```python
from build123d import *

# Parameters (mm, degrees)
SKETCH1_W           = 40
SKETCH1_H           = 30
BOSS_EXTRUDE1_DEPTH = 2
SKETCH2_W           = 20
SKETCH2_H           = 30
BOSS_EXTRUDE2_DEPTH = 2
SKETCH3_W           = 20
SKETCH3_H           = 30
BOSS_EXTRUDE3_DEPTH = 2
SKETCH5_R           = 5
CUT_EXTRUDE2_DEPTH  = 55.595167513


with BuildPart() as part:
    # Sketch1 → Boss-Extrude1 (new body)
    with BuildSketch(Plane.XY):
        with Locations((-21.168831169, 10.38961039)):
            Rectangle(SKETCH1_W, SKETCH1_H)
    extrude(amount=BOSS_EXTRUDE1_DEPTH)

    # Sketch2 → Boss-Extrude2 (add)
    with BuildSketch(Plane.ZY.offset(41.168831169)):
        with Locations((10, 10.38961039)):
            Rectangle(SKETCH2_W, SKETCH2_H)
    extrude(amount=BOSS_EXTRUDE2_DEPTH)

    # Sketch3 → Boss-Extrude3 (add)
    with BuildSketch(Plane(origin=(-1.168831169, 0, 0), x_dir=(0, 0, -1), z_dir=(1, 0, 0))):
        with Locations((-10, 10.38961039)):
            Rectangle(SKETCH3_W, SKETCH3_H)
    extrude(amount=BOSS_EXTRUDE3_DEPTH)

    # Sketch5 → Cut-Extrude2 (cut, through all)
    with BuildSketch(Plane(origin=(0.831168831, 0, 0), x_dir=(0, 0, -1), z_dir=(1, 0, 0))):
        with Locations(Location((-10, 10.38961039, 0), (0, 0, 90))):
            Circle(SKETCH5_R)
    extrude(amount=-CUT_EXTRUDE2_DEPTH, mode=Mode.SUBTRACT)


solid = part.part
```
Model file for the job. Use its own axes, mm. A direction names the side the tool comes from. Give positions to 0.01 mm unless a question says otherwise; leave off trailing zeros. Write each loop counter-clockwise with the first axis right and the second up, starting at its lowest first coordinate (ties: lowest second). Pieces come first, ordered by that corner, then holes. Notation, with made-up numbers: M -1.5,4.25 L 35.5,4.25 A17 cw 35.5,36.25 Z; hole C 83.25,45 d9. An arc over 180 degrees is marked long. Use a Markdown table: item, result.
1) Cut at D-D (y = 23.75). List the corners of the cut face in (x, z).
Responses:
| item | result |
|---|---|
| outline | M -43.17,0 L 0.83,0 L 0.83,20 L -1.17,20 L -1.17,2 L -41.17,2 L -41.17,20 L -43.17,20 Z |
2) Drill centre lines: line 1 (X direction, y = 15.75, z = 18.75); line 2 (Z direction, x = -41, y = 11.5). Where is each one in solid material? Low to high. Write a range as from..to.
Responses:
| item | result |
|---|---|
| line 1 | x = -43.17..-41.17, -1.17..0.83 |
| line 2 | z = 0..2 |
3) Cut at B-B (y = 7.75). List the corners of the cut face in (x, z), and give its area (3 significant figures).
Responses:
| item | result |
|---|---|
| outline | M -43.17,0 L 0.83,0 L 0.83,5.75 L -1.17,5.75 L -1.17,2 L -41.17,2 L -41.17,5.75 L -43.17,5.75 Z; M -43.17,14.25 L -41.17,14.25 L -41.17,20 L -43.17,20 Z; M -1.17,14.25 L 0.83,14.25 L 0.83,20 L -1.17,20 Z |
| area | 126 mm2 |
4) Cut at A-A (z = 10). List the corners of the cut face in (x, y).
Responses:
| item | result |
|---|---|
| outline | M -43.17,-4.61 L -41.17,-4.61 L -41.17,5.39 L -43.17,5.39 Z; M -43.17,15.39 L -41.17,15.39 L -41.17,25.39 L -43.17,25.39 Z; M -1.17,-4.61 L 0.83,-4.61 L 0.83,5.39 L -1.17,5.39 Z; M -1.17,15.39 L 0.83,15.39 L 0.83,25.39 L -1.17,25.39 Z |
5) Pull direction X, two halves, no side cores. Call faces 3 (the flat face through (0.831, 7, 6)), 4 (the flat face through (-21, 11, 2)), 5 (the flat face through (-1.169, 7, 15)), 6 (the flat face through (0, 10, 20)): +X half, -X half, draft (parallel to the pull), parting line (faces both ways), or undercut.
Responses:
| item | result |
|---|---|
| face 3 | +X half |
| face 4 | undercut |
| face 5 | undercut |
| face 6 | draft |
6) Tool access for faces 1 (the flat face through (-42, 10, 20)), 2 (the flat face through (-41.169, 7, 15)): list every direction of +Z, -Z, +X, -X, +Y, -Y with a clear straight run to the whole face (end or side of a thin tool).
Responses:
| item | result |
|---|---|
| face 1 | +Z, +X, -X, +Y, -Y |
| face 2 | +Z, +Y, -Y |
7) Cut at C-C (z = 2.5). List the corners of the cut face in (x, y).
Responses:
| item | result |
|---|---|
| outline | M -43.17,-4.61 L -41.17,-4.61 L -41.17,25.39 L -43.17,25.39 Z; M -1.17,-4.61 L 0.83,-4.61 L 0.83,25.39 L -1.17,25.39 Z |
8) Pin check, flat tip, straight feed: pin 1 (2 mm diameter, centred on x = -22, y = 18.5, fed in from +Z). Stop position of the tip, or through.
Responses:
| item | result |
|---|---|
| pin 1 | stops at z = 2 |
